Can you work these out from the model? Positions are in its coordinate system, mm. A direction names the side the tool comes from. Give positions to 0.01 mm unless a question says otherwise; leave off trailing zeros. Loops run counter-clockwise (first coordinate to the right, second up) from the corner with the lowest first, then second, coordinate; pieces in that order, holes last. Notation, with made-up numbers: (73.25, 36.5) -> (100.25, 36.5) arc R30 cw to (100.25, 68.5) -> close; hole circle Ø2 at (-19, 86.25). An arc over 180 degrees is marked (long way). Return JSON: item names as keys, results as strings. Group by question number.
Q1. I need wall thicknesses on line 1 along X through (y, z) = (-11.5, -40); line 2 along Z through (x, y) = (89, 20) (3 decimals); line 3 along Y through (x, z) = (-29, -5.5) (3 decimals). Which ranges of each line are inside material? Lowest first, please. Write a range as [from, to].
Q2. Thinking about a two-plate mould opening in X: for faces 4 (the flat face through (126, 25.4, 0)), 5 (the flat face through (125, 1, -3.175)), 6 (the flat face through (254, 1, -25)), 7 (the flat face through (304.8, 0, -22)), which applies, pulls with the +X half, pulls with the -X half, needs draft (parallel to the pull), parting line crosses it, or undercut?
Q3. Will these pins go through, and if not, where does the flat tip stop? pin 1 (5 mm diameter, centred on x = 167.5, y = -8, fed in from -Z) (3 decimals); pin 2 (22 mm diameter, centred on x = -13.5, z = -35.5, fed in from -Y) (3 decimals).
Q4. Suppose I cut it at C-C, the plane x = 274. Please give me the cut outline in (y, z) (3 decimals).
Q5. Suppose I cut it at B-B, the plane y = 6. Please give me the cut outline in (x, z) (3 decimals), and give its area (3 significant figures).
Q6. Suppose I cut it at A-A, the plane z = -14.5. Please give me the cut outline in (x, y) (3 decimals), and give its area (3 significant figures).
Q7. Which directions (+Z, -Z, +X, -X, +Y, -Y) give clear straight access to the entire face, cutting with the end or side of a thin tool? Please do faces 1 (the flat face through (0, 2, -25)), 2 (the flat face through (-25, -22.225, -26)), 3 (the flat face through (279, 1, -47.625)).
```python
from build123d import *

# Parameters (mm, degrees)
F0_W     = 50.8
F0_H     = 6.35
F1_DEPTH = 254
F2_R     = 3.17499
F3_W     = 47.625
F3_H     = 50.8
F4_DEPTH = 50.8
F6_DEPTH = 50.8
F8_DEPTH = 50.8


# Not quite as in the source:
# - a fillet or chamfer is up to 0.001 mm smaller than in the source, because OpenCascade refuses the exact size


with BuildPart() as f1:
    # F0 (on Right) → F1 (new body)
    with BuildSketch(Plane.YZ):
        Rectangle(F0_W, F0_H)
    extrude(amount=F1_DEPTH)

    # F2 (radius 3.175 in the source; OpenCascade refuses exactly that, so slightly less here)
    f2_edges = [f1.edges().sort_by_distance(p)[0] for p in [
        (127, -25.4, 3.175),
        (127, -25.4, -3.175),
    ]]
    fillet(f2_edges, radius=F2_R)

    # F3 (on face) → F4 (join)
    with BuildSketch(Plane(origin=(0, 0, 0), x_dir=(0, -1, 0), z_dir=(-1, 0, 0))):
        with Locations((-1.5875, -22.225)):
            Rectangle(F3_W, F3_H)
    extrude(amount=F4_DEPTH)

    # F5 (on face) → F6 (join, through all)
    with BuildSketch(Plane(origin=(0, 0, 0), x_dir=(0, -1, 0), z_dir=(-1, 0, 0))):
        with BuildLine():
            Line((22.225, 3.175), (22.225, -3.175))
            ThreePointArc((22.225, -3.175), (25.4, 0), (22.225, 3.175))
        make_face()
    extrude(amount=F6_DEPTH)

    # F7 (on face) → F8 (join)
    with BuildSketch(Plane.YZ.offset(254)):
        with BuildLine():
            Line((-22.225, -3.175), (-22.225, -47.625))
            Line((-22.225, -47.625), (25.4, -47.625))
            Line((25.4, -47.625), (25.4, 3.175))
            Line((25.4, 3.175), (-22.225, 3.175))
            ThreePointArc((-22.225, 3.175), (-25.4, 0), (-22.225, -3.175))
        make_face()
    extrude(amount=F8_DEPTH)


solid = f1.part
```
Ans:
{
 "1": {"line 1": "x = [-50.8, 0], [254, 304.8]", "line 2": "z = [-3.175, 3.175]", "line 3": "y = [-22.225, 25.4]"},
 "2": {"face 4": "needs draft", "face 5": "undercut", "face 6": "undercut", "face 7": "pulls with the +X half"},
 "3": {"pin 1": "stops at z = -3.175", "pin 2": "stops at y = -22.225"},
 "4": {"outline": "(-22.225, -47.625) -> (25.4, -47.625) -> (25.4, 3.175) -> (-22.225, 3.175) arc R3.175 ccw to (-22.225, -3.175) -> close"},
 "5": {"outline": "(-50.8, -47.625) -> (0, -47.625) -> (0, -3.175) -> (254, -3.175) -> (254, -47.625) -> (304.8, -47.625) -> (304.8, 3.175) -> (-50.8, 3.175) -> close", "area": "6,770 mm^2"},
 "6": {"outline": "(-50.8, -22.225) -> (0, -22.225) -> (0, 25.4) -> (-50.8, 25.4) -> close; (254, -22.225) -> (304.8, -22.225) -> (304.8, 25.4) -> (254, 25.4) -> close", "area": "4,840 mm^2"},
 "7": {"face 1": "-Z, +Y, -Y", "face 2": "-Z, +X, -X, -Y", "face 3": "-Z, +X, -X, +Y, -Y"}
}
